from build123d import *

# Parameters (mm, degrees)
SKETCH1_W                = 47
SKETCH1_H                = 22
SKETCH1_R                = 1.55
BOSS_EXTRUDE1_DEPTH      = 1.6
FILLET1_R                = 3.1
BOSS_EXTRUDE4_DEPTH      = 0.1
BOSS_EXTRUDE4_DEPTH_BACK = 1.7
SKETCH2_R                = 3
SKETCH2_R_2              = 1.55
SKETCH3_R                = 7.75
BOSS_EXTRUDE8_DEPTH      = 11


with BuildPart() as part:
    # Sketch1 → Boss-Extrude1 (new body)
    with BuildSketch(Plane.XY):
        Rectangle(SKETCH1_W, SKETCH1_H)
        with Locations((-20, 7.5)):
            Circle(SKETCH1_R, mode=Mode.SUBTRACT)
        with Locations((20, 7.5)):
            Circle(SKETCH1_R, mode=Mode.SUBTRACT)
        with Locations((20, -7.5)):
            Circle(SKETCH1_R, mode=Mode.SUBTRACT)
        with Locations((-20, -7.5)):
            Circle(SKETCH1_R, mode=Mode.SUBTRACT)
    extrude(amount=BOSS_EXTRUDE1_DEPTH)

    # Fillet1
    fillet1_edges = [part.edges().sort_by_distance(p)[0] for p in [
        (23.5, -11, 0.8),
        (-23.5, -11, 0.8),
        (-23.5, 11, 0.8),
        (23.5, 11, 0.8),
    ]]
    fillet(fillet1_edges, radius=FILLET1_R)

    # Sketch2 → Boss-Extrude4 (add, two sides: drawn at the far end of the back side and taken through both)
    # profile 1 of 4: a face of its own
    with BuildSketch(Plane.XY.offset(1.6).offset(-BOSS_EXTRUDE4_DEPTH_BACK)):
        with Locations((-20, 7.5)):
            Circle(SKETCH2_R)
        with Locations((-20, 7.5)):
            Circle(SKETCH2_R_2, mode=Mode.SUBTRACT)
    # profile 2 of 4: a face of its own
    with BuildSketch(Plane.XY.offset(1.6).offset(-BOSS_EXTRUDE4_DEPTH_BACK)):
        with Locations((-20, -7.5)):
            Circle(SKETCH2_R)
        with Locations((-20, -7.5)):
            Circle(SKETCH2_R_2, mode=Mode.SUBTRACT)
    # profile 3 of 4: a face of its own
    with BuildSketch(Plane.XY.offset(1.6).offset(-BOSS_EXTRUDE4_DEPTH_BACK)):
        with Locations((20, 7.5)):
            Circle(SKETCH2_R)
        with Locations((20, 7.5)):
            Circle(SKETCH2_R_2, mode=Mode.SUBTRACT)
    # profile 4 of 4: a face of its own
    with BuildSketch(Plane.XY.offset(1.6).offset(-BOSS_EXTRUDE4_DEPTH_BACK)):
        with Locations((20, -7.5)):
            Circle(SKETCH2_R)
        with Locations((20, -7.5)):
            Circle(SKETCH2_R_2, mode=Mode.SUBTRACT)
    extrude(amount=BOSS_EXTRUDE4_DEPTH + BOSS_EXTRUDE4_DEPTH_BACK)

    # Sketch3 → Boss-Extrude8 (add)
    with BuildSketch(Plane.XY.offset(1.6)):
        with Locations(Location((11.5, 0, 0), (0, 0, 180))):
            Circle(SKETCH3_R)
        with Locations(Location((-11.5, 0, 0), (0, 0, 180))):
            Circle(SKETCH3_R)
    extrude(amount=BOSS_EXTRUDE8_DEPTH)


solid = part.part
Design review of the part built by this model. Coordinates are the model's own, in mm. A direction names the side the tool comes from. Coordinates: 2 decimals unless noted, no trailing zeros. Order: outer loops, then holes, each group sorted by start corner. A loop starts at its lowest first (then second) coordinate and runs counter-clockwise, first axis right, second up. Notation, with made-up numbers: M 51,-33 L 89,-33 A29 ccw 89,6 Z; hole C 89.25,11.5 d8. An arc over 180 degrees is marked long. Use a Markdown table: item, result.
(1) Add section D-D (y = -6.5). Count the separate pieces of the cut face and the enclosed holes in it, then the cut area to 3 significant figures.
Worked answers:
| item | result |
|---|---|
| separate pieces | 3 |
| enclosed holes | 0 |
| area | 255 mm2 |
(2) Draft analysis for pull direction Y (two halves, no side actions). For faces 6 (the flat face through (-19, 6, -0.1)), 7 (the flat face through (0, 11, 1)), 8 (the cylindrical face through (-3.757, -0.341, 7.023)), 9 (the cylindrical face through (-18.568, -8.094, 0.787)), state which applies: released by +Y, released by -Y, zero draft, split by the parting line, or undercut.
Worked answers:
| item | result |
|---|---|
| face 6 | zero draft |
| face 7 | released by +Y |
| face 8 | split by the parting line |
| face 9 | undercut |
(3) Wall thickness on probe 1 along Y at (x, z) = (-20, 1.1); probe 2 along X at (y, z) = (0.25, 7.75); probe 3 along Z at (x, y) = (8.5, -5.75): over which ranges is each line inside the solid? List them lowest first.
Worked answers:
| item | result |
|---|---|
| probe 1 | y = -11 to -9.05, -5.95 to 5.95, 9.05 to 11 |
| probe 2 | x = -19.25 to -3.75, 3.75 to 19.25 |
| probe 3 | z = 0 to 12.6 |
(4) For faces 1 (the flat face through (21, 6, 1.7)), 2 (the flat face through (-19, -9, 1.7)), 3 (the cylindrical face through (19.243, -0.341, 7.023)), 4 (the flat face through (21, -9, 1.7)), 5 (the flat face through (-19, 6, 1.7)), list the 3-axis set-ups (+Z, -Z, +X, -X, +Y, -Y) from which the entire face can be reached by the end or side of a thin tool; tool diameter is ignored.
Worked answers:
| item | result |
|---|---|
| face 1 | +Z, +X, +Y |
| face 2 | +Z, -X, -Y |
| face 3 | +Z |
| face 4 | +Z, +X, -Y |
| face 5 | +Z, -X, +Y |
(5) For P1, Ø6, axis at y = -3.5, z = 8.5, coming from the -X side; P2, Ø5, axis at x = -2.5, z = 11.5, coming from the +Y side; P3, Ø1.8, axis at x = 19, y = 8.5, coming from the +Z side; P4, Ø1.9, axis at x = 20, y = 7.5, coming from the +Z side, all flat-tipped, find the tip position at first contact; note any pin that passes through.
Worked answers:
| item | result |
|---|---|
| P1 | stops at x = -19.23 |
| P2 | stops at y = 4.22 |
| P3 | stops at z = 1.7 |
| P4 | passes through |
(6) Add section C-C (y = 0). Give the boundary of the cut face in (x, z).
Worked answers:
| item | result |
|---|---|
| outline | M -23.5,0 L 23.5,0 L 23.5,1.6 L 19.25,1.6 L 19.25,12.6 L 3.75,12.6 L 3.75,1.6 L -3.75,1.6 L -3.75,12.6 L -19.25,12.6 L -19.25,1.6 L -23.5,1.6 Z |
(7) Add section A-A (x = 11.5). Give the boundary of the cut face in (y, z), then the cut area to 3 significant figures.
Worked answers:
| item | result |
|---|---|
| outline | M -11,0 L 11,0 L 11,1.6 L 7.75,1.6 L 7.75,12.6 L -7.75,12.6 L -7.75,1.6 L -11,1.6 Z |
| area | 206 mm2 |
(8) Add section B-B (z = 4). Give the boundary of the cut face in (x, y), then the cut area to 3 significant figures.
Worked answers:
| item | result |
|---|---|
| outline | C -11.5,0 d15.5; C 11.5,0 d15.5 |
| area | 377 mm2 |
